from build123d import *

# Parameters (mm, degrees)
HOLE_WIZARD_M3_1_D = 2.5
CHAMFER_1_SIZE     = 0.5


with BuildPart() as part:
    # 草图1 → 旋转1 (revolve)
    with BuildSketch(Plane(origin=(0, 0, 0), x_dir=(0, 0, -1), z_dir=(1, 0, 0))):
        Polygon((2.75, 0), (10, 0), (10, 2), (4.5, 2), (4.5, 4.5), (2.75, 4.5), (2.75, 1), (1, 1), (1, 0), align=None)
    revolve(axis=Axis((0, 0, 0), (0, 1, 0)))

    # M3 螺纹孔的螺纹孔钻头1 (through all)
    with Locations(Plane(origin=(0, 2, 0), x_dir=(1, 0, 0), z_dir=(0, 1, 0))):
        with Locations((0, -7), (0, 7), (-7, 0), (7, 0)):
            Hole(HOLE_WIZARD_M3_1_D / 2)

    # 倒角1
    chamfer_1_edges = [part.edges().sort_by_distance(p)[0] for p in [
        (0, 4.5, 2.75),
    ]]
    chamfer(chamfer_1_edges, length=CHAMFER_1_SIZE)


solid = part.part
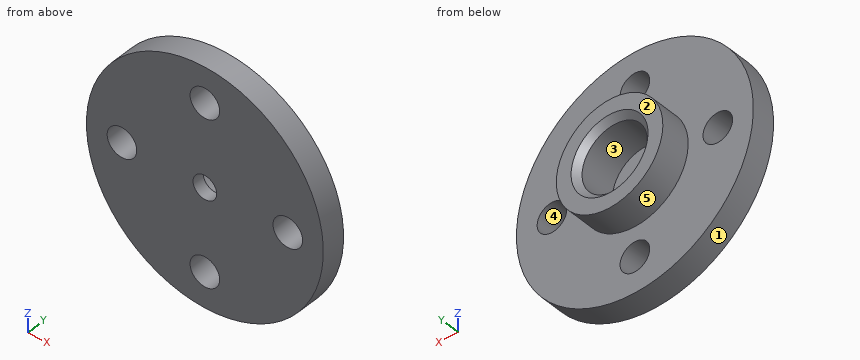
Geometry: final body of the model. Coordinates: model frame, mm. Face numbers are marked on the shaded views. A direction names the side the tool comes from. Coordinates: 2 decimals unless noted, no trailing zeros. Loops run counter-clockwise (first coordinate to the right, second up) from the corner with the lowest first, then second, coordinate; pieces in that order, holes last. Notation, with made-up numbers: M 77,6 L 83,6 A6 ccw 83,14 Z; hole C -16.75,-20 d5. An arc over 180 degrees is marked long. One line per item, written item: value. Start each with the question number.
1) Pin query (flat end, axial travel): P1, Ø6, axis at x = -0.5, z = -0.5, coming from the +Y side; P2, Ø2, axis at x = 0, z = 7, coming from the -Y side; P3, Ø1, axis at x = 8, y = 0.5, coming from the -Z side. Return the tip coordinate at first contact, or that it passes through.
2) Cut plane C-C (y = 0.65). Return loops of the section in (x, z), then the cut area to 3 significant figures.
3) Cut plane B-B (x = 0). Return loops of the section in (y, z).
4) Material intervals for L1, parallel to Z at x = 0, y = 1.35; L2, parallel to Z at x = -0.5, y = 1.05; L3, parallel to Y at x = -0.5, z = -5, sorted ascending. Write a range as from..to.
5) Draft query along X for the marked faces 1, 2 and 3. Return one class per face: released by +X, released by -X, zero draft, split by the parting line, or undercut.
6) Cut plane D-D (x = 6.5). Return loops of the section in (y, z).
7) Cut plane A-A (z = 0). Return loops of the section in (x, y), then the cut area to 3 significant figures.
8) Reachability of the marked faces 4 and 5 from +Z, -Z, +X, -X, +Y, -Y: full face, straight path, thin tool, end or side. Return the list, or none.
Evaluation:
1. P1: y = 4.5
1. P2: through
1. P3: z = -6.61
2. outline: C 0,0 d20; hole C -7,0 d2.5; hole C 0,-7 d2.5; hole C 0,7 d2.5; hole C 0,0 d2; hole C 7,0 d2.5
2. area: 291 mm^2
3. outline: M 0,-10 L 2,-10 L 2,-8.25 L 0,-8.25 Z; M 0,-5.75 L 2,-5.75 L 2,-4.5 L 4.5,-4.5 L 4.5,-3.25 L 4,-2.75 L 1,-2.75 L 1,-1 L 0,-1 Z; M 0,1 L 1,1 L 1,2.75 L 4,2.75 L 4.5,3.25 L 4.5,4.5 L 2,4.5 L 2,5.75 L 0,5.75 Z; M 0,8.25 L 2,8.25 L 2,10 L 0,10 Z
4. L1: -10..-8.25, -5.75..-2.75, 2.75..5.75, 8.25..10
4. L2: -9.99..-8.15, -5.85..-2.7, 2.7..5.85, 8.15..9.99
4. L3: 0..2
5. face 1: split by the parting line
5. face 2: zero draft
5. face 3: undercut
6. outline: M 0,-7.6 L 2,-7.6 L 2,-1.15 L 0,-1.15 Z; M 0,1.15 L 2,1.15 L 2,7.6 L 0,7.6 Z
7. outline: M -10,0 L -8.25,0 L -8.25,2 L -10,2 Z; M -5.75,0 L -1,0 L -1,1 L -2.75,1 L -2.75,4 L -3.25,4.5 L -4.5,4.5 L -4.5,2 L -5.75,2 Z; M 1,0 L 5.75,0 L 5.75,2 L 4.5,2 L 4.5,4.5 L 3.25,4.5 L 2.75,4 L 2.75,1 L 1,1 Z; M 8.25,0 L 10,0 L 10,2 L 8.25,2 Z
7. area: 31.0 mm^2
8. face 4: +Y, -Y
8. face 5: +Y
